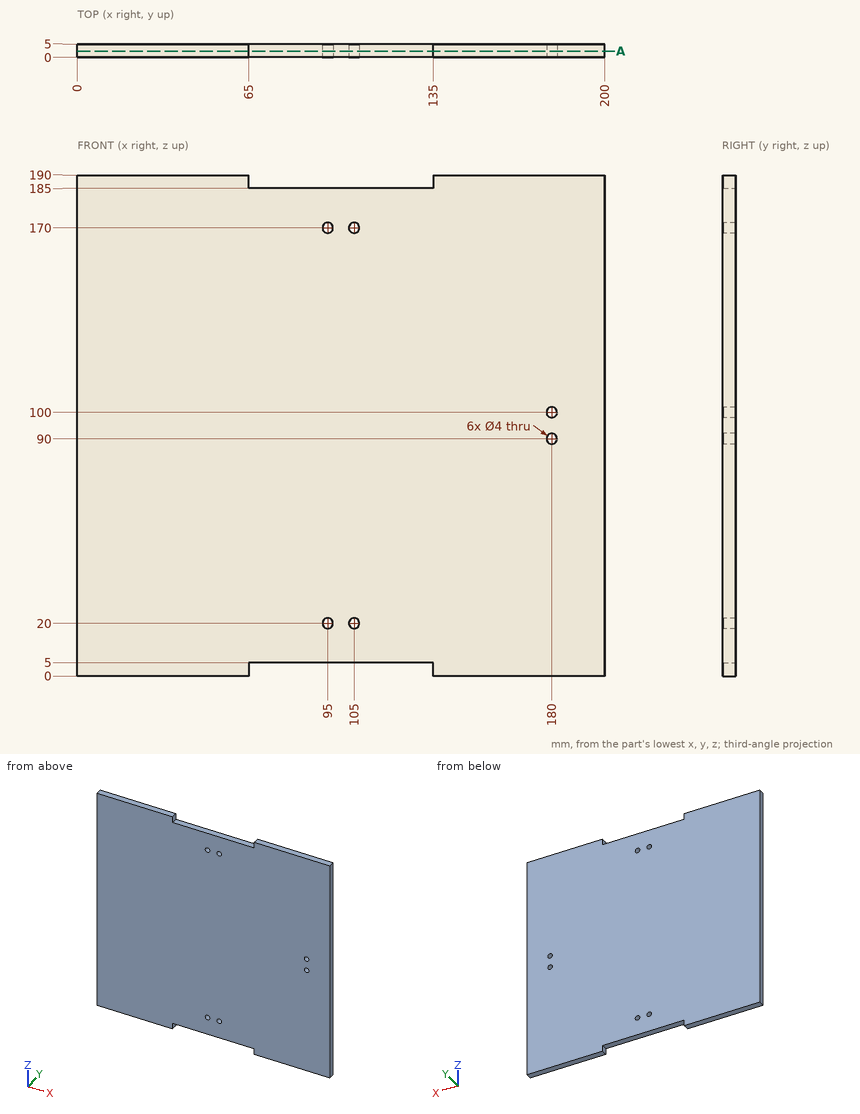
Job drawing, mm, ordinate dimensions from the low corner. One solid piece. Coordinates: 2 decimals unless noted, no trailing zeros. Loops run counter-clockwise (first coordinate to the right, second up) from the corner with the lowest first, then second, coordinate; pieces in that order, holes last. Notation, with made-up numbers: (37, -35) - (89, -35) arc R24 ccw to (89, -8) - close; hole circle Ø2 at (80, -23). An arc over 180 degrees is marked (long way). Write item = value, one per line. Start each with the question number.
Q1. Cut at A-A, the plane y = 2.3. List the corners of the cut face in (x, z), then the cut area to 3 significant figures.
Q2. Drill centre lines: L1, parallel to Z at x = 95, y = 3.45; L2, parallel to X at y = 2.85, z = 170; L3, parallel to Z at x = 180, y = 1. Where is each one in solid material? Low to high.
Q3. Flat gauge pins, fed straight in: pin 1 Ø3.5 at (x, z) = (180, 100) entering from +Y; pin 2 Ø1.5 at (x, y) = (84.5, 2.5) entering from +Z. Where does each tip first touch, or does it go through?
Computed:
q1.outline = (0, 0) - (65, 0) - (65, 5) - (135, 5) - (135, 0) - (200, 0) - (200, 190) - (135, 190) - (135, 185) - (65, 185) - (65, 190) - (0, 190) - close; hole circle Ø4 at (95, 20); hole circle Ø4 at (95, 170); hole circle Ø4 at (105, 20); hole circle Ø4 at (105, 170); hole circle Ø4 at (180, 90); hole circle Ø4 at (180, 100)
q1.area = 37,200 mm²
q2.L1 = 5 to 18, 22 to 168, 172 to 185
q2.L2 = 0 to 93, 97 to 103, 107 to 200
q2.L3 = 0 to 88, 92 to 98, 102 to 190
q3.pin_1 = through
q3.pin_2 = 185
